```python
from build123d import *

# Parameters (mm, degrees)
F0_R     = 3
F1_DEPTH = 4.5
F0_R_2   = 6.35
F2_DEPTH = 1.5
F3_DEPTH = 25
F4_R     = 0.3
F5_R     = 4
F6_DEPTH = 1
F7_SIZE  = 0.2


with BuildPart() as f1:
    # F0 (on Top) → F1 (new body)
    with BuildSketch(Plane.XY):
        Polygon((2.921558, -4.912687), (5.715291, 0.0738), (2.793733, 4.986487), (-2.921558, 4.912687), (-5.715291, -0.0738), (-2.793733, -4.986487), align=None)
        Circle(F0_R, mode=Mode.SUBTRACT)
        Circle(F0_R)
    extrude(amount=F1_DEPTH)

    # F0 (on Top) → F2 (join)
    with BuildSketch(Plane.XY):
        Circle(F0_R_2)
        Polygon((2.793733, 4.986487), (5.715291, 0.0738), (2.921558, -4.912687), (-2.793733, -4.986487), (-5.715291, -0.0738), (-2.921558, 4.912687), align=None, mode=Mode.SUBTRACT)
        Circle(F0_R)
        Polygon((2.921558, -4.912687), (5.715291, 0.0738), (2.793733, 4.986487), (-2.921558, 4.912687), (-5.715291, -0.0738), (-2.793733, -4.986487), align=None)
        Circle(F0_R, mode=Mode.SUBTRACT)
    extrude(amount=-F2_DEPTH)

    # F0 (on Top) → F3 (join)
    with BuildSketch(Plane.XY):
        Circle(F0_R)
    extrude(amount=-F3_DEPTH)

    # F4
    f4_edges = [f1.edges().sort_by_distance(p)[0] for p in [
        (6.35, 0, -0.75),
        (-6.35, 0, 0),
        (-6.35, 0, -1.5),
    ]]
    fillet(f4_edges, radius=F4_R)

    # F5 (on face) → F6 (cut)
    with BuildSketch(Plane.XY.offset(4.5)):
        Circle(F5_R)
    extrude(amount=-F6_DEPTH, mode=Mode.SUBTRACT)

    # F7
    f7_edges = [f1.edges().sort_by_distance(p)[0] for p in [
        (0.063913, -4.949587, 4.5),
        (-4.254512, -2.530144, 4.5),
        (4.318425, -2.419444, 4.5),
        (-4.318425, 2.419444, 4.5),
        (4.254512, 2.530144, 4.5),
        (-0.063913, 4.949587, 4.5),
        (-4, 0, 4.5),
    ]]
    chamfer(f7_edges, length=F7_SIZE)


solid = f1.part
```
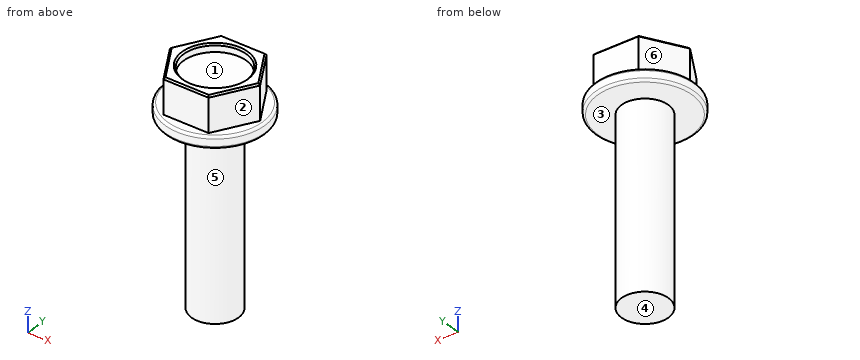
The model under review builds one solid part; all positions refer to its coordinate system, in mm. Face numbers are marked on the shaded views. A direction names the side the tool comes from. Round coordinates to 2 decimals unless told otherwise and drop trailing zeros. Order: outer loops, then holes, each group sorted by start corner. A loop starts at its lowest first (then second) coordinate and runs counter-clockwise, first axis right, second up.
Item 1: For pin 1 (2 mm diameter, centred on x = 0, z = -6, fed in from -Y); pin 2 (5 mm diameter, centred on y = 0.5, z = -20.5, fed in from -X); pin 3 (1 mm diameter, centred on y = 3, z = -20, fed in from -X), all flat-tipped, find the tip position at first contact; note any pin that passes through.
Working result:
pin 1: stops at y = -3
pin 2: stops at x = -3
pin 3: stops at x = -1.66
Item 2: Machinability: for the marked faces 4, 5 and 6, which of the approach directions +Z, -Z, +X, -X, +Y, -Y give a long, thin tool a straight path to every point of the face, cutting with its end or side? Answer none if there is none.
Working result:
face 4: -Z, +X, -X, +Y, -Y
face 5: -Z
face 6: +Z, -X, +Y
Item 3: Draft analysis for pull direction X (two halves, no side actions). For the marked faces 1, 2 and 3, state which applies: released by +X, released by -X, zero draft, split by the parting line, or undercut.
Working result:
face 1: undercut
face 2: released by +X
face 3: zero draft
Item 4: To check wall thickness, follow probe 1 along Z at (x, y) = (4.5, -1.25); probe 2 along Z at (x, y) = (3.25, 4.75); probe 3 along Y at (x, z) = (0, 3.7). State the ranges of each line that lie inside material, in increasing order.
Working result:
probe 1: z = -1.5 to 4.5
probe 2: z = -1.5 to 0
probe 3: y = -4.95 to -4, 4 to 4.95
Item 5: Add section B-B, the plane x = 0. State the section outline as (y, z) points.
Working result:
outline: (-6.35, -1.2) arc R0.3 ccw to (-6.05, -1.5) - (-3, -1.5) - (-3, -25) - (3, -25) - (3, -1.5) - (6.05, -1.5) arc R0.3 ccw to (6.35, -1.2) - (6.35, -0.3) arc R0.3 ccw to (6.05, 0) - (4.95, 0) - (4.95, 4.3) - (4.75, 4.5) - (4.2, 4.5) - (4, 4.3) - (4, 3.5) - (-4, 3.5) - (-4, 4.3) - (-4.2, 4.5) - (-4.75, 4.5) - (-4.95, 4.3) - (-4.95, 0) - (-6.05, 0) arc R0.3 ccw to (-6.35, -0.3) - close
Item 6: Add section A-A, the plane z = -18.25. State the section outline as (x, y) points.
Working result:
outline: circle Ø6 at (0, 0)
